Part model, mm, in its own coordinate system. A direction names the side the tool comes from. Round coordinates to 2 decimals unless told otherwise and drop trailing zeros. Loops run counter-clockwise (first coordinate to the right, second up) from the corner with the lowest first, then second, coordinate; pieces in that order, holes last. Notation, with made-up numbers: M 63.5,67 L 94.5,67 A21 ccw 94.5,106 Z; hole C -35.75,5.25 d2. An arc over 180 degrees is marked long. Put each result on its own line as item: value. Start each with the question number.
1) Pull direction Y, two halves, no side cores. Call faces 6 (the cylindrical face through (-0.495, -97.905, 0.21)), 7 (the cylindrical face through (-8.337, -54.779, -3.07)), 8 (the flat face through (26, -105.4, 0)): +Y half, -Y half, draft (parallel to the pull), parting line (faces both ways), or undercut.
2) Slice it at A-A on y = 0. Give the cut face in (x, z).
3) Probe line 1 along Y through (x, z) = (0.5, 5.5); line 2 along Y through (x, z) = (1, 8); line 3 along Z through (x, y) = (-30, -117). List the from-to ranges inside material, lowest first.
4) Drop flat-ended pins along their axis: pin 1 Ø16 at (x, y) = (-3.5, -47) entering from -Z; pin 2 Ø6 at (x, y) = (1.5, -45.5) entering from +Z; pin 3 Ø1.5 at (y, z) = (-23, 6.5) entering from +X; pin 4 Ø11 at (x, y) = (0, 0) entering from +Z. Give the stop position or say it passes through.
5) Which spindle directions (+Z, -Z, +X, -X, +Y, -Y) get a long thin tool onto all of the face, cutting with end or side? Do faces 1 (the flat face through (30, -117.4, 9)), 2 (the flat face through (-30, -117.4, 9)), 3 (the cylindrical face through (9.444, -53.631, 6.93)), 4 (the cylindrical face through (-35, -111, 0)), 5 (the flat face through (0, -62, -2.5)). Say none if no direction does.
```python
from build123d import *

# Parameters (mm, degrees)
SKETCH2_R           = 12.5
SKETCH2_R_2         = 9
BOSS_EXTRUDE1_DEPTH = 10
BOSS_EXTRUDE2_DEPTH = 15
BOSS_EXTRUDE3_DEPTH = 7.5
CUT_EXTRUDE2_START  = 7.5
CUT_EXTRUDE2_DEPTH  = 5
BOSS_EXTRUDE8_REACH = 149.366
BOSS_EXTRUDE8_START = 12
SKETCH4_R           = 3.25
SKETCH4_14_R        = 3.25
CUT_EXTRUDE3_DEPTH  = 136.366207009
FILLET1_R           = 2
FILLET5_R           = 2


with BuildPart() as part:
    # Sketch2 → Boss-Extrude1 (new, symmetric)
    with BuildSketch(Plane.XY):
        Circle(SKETCH2_R)
        Circle(SKETCH2_R_2, mode=Mode.SUBTRACT)
    extrude(amount=BOSS_EXTRUDE1_DEPTH, both=True)



with BuildPart() as body_2:
    # Sketch2_3 → Boss-Extrude2 (new, symmetric)
    with BuildSketch(Plane.XY):
        with BuildLine():
            ThreePointArc((15.952867936, -100.506382817), (8.454666221, -96.342389581), (0, -94.9))
            Line((0, -94.9), (0, -97.9))
            ThreePointArc((0, -97.9), (15.909902577, -104.490097423), (22.5, -120.4))
            Line((22.5, -120.4), (35, -120.4))
            Line((35, -120.4), (35, -117.4))
            Line((35, -117.4), (25.322914524, -117.4))
            ThreePointArc((25.322914524, -117.4), (22.299576897, -108.031537274), (15.952867936, -100.506382817))
        make_face()
        with BuildLine():
            Line((0, -97.9), (0, -94.9))
            ThreePointArc((0, -94.9), (-8.454666221, -96.342389581), (-15.952867936, -100.506382817))
            ThreePointArc((-15.952867936, -100.506382817), (-22.299576897, -108.031537274), (-25.322914524, -117.4))
            Line((-25.322914524, -117.4), (-35, -117.4))
            Line((-35, -117.4), (-35, -120.4))
            Line((-35, -120.4), (-22.5, -120.4))
            ThreePointArc((-22.5, -120.4), (-15.909902577, -104.490097423), (0, -97.9))
        make_face()
    extrude(amount=BOSS_EXTRUDE2_DEPTH, both=True)


with BuildPart() as part_1:
    add(part.part)

    add(body_2.part)  # Boss-Extrude3 merges body 2
    # Sketch2_4 → Boss-Extrude3 (add, symmetric)
    with BuildSketch(Plane.XY):
        with BuildLine():
            Line((0, -94.9), (0, -12.5))
            ThreePointArc((0, -12.5), (-4.253905297, -11.753905297), (-8, -9.604686356))
            Line((-8, -9.604686356), (-15.952867936, -100.506382817))
            ThreePointArc((-15.952867936, -100.506382817), (-8.454666221, -96.342389581), (0, -94.9))
        make_face()
        with BuildLine():
            ThreePointArc((8, -9.604686356), (4.253905297, -11.753905297), (0, -12.5))
            Line((0, -12.5), (0, -94.9))
            ThreePointArc((0, -94.9), (8.454666221, -96.342389581), (15.952867936, -100.506382817))
            Line((15.952867936, -100.506382817), (8, -9.604686356))
        make_face()
    extrude(amount=BOSS_EXTRUDE3_DEPTH, both=True)

    # Sketch3 → Cut-Extrude2 (cut)
    with BuildSketch(Plane.XY.offset(CUT_EXTRUDE2_START)):
        with BuildLine():
            Line((-5.4187458, -14.521955583), (-12.438451255, -94.757556076))
            ThreePointArc((-12.438451255, -94.757556076), (0, -91.9), (12.438451255, -94.757556076))
            Line((12.438451255, -94.757556076), (5.4187458, -14.521955583))
            ThreePointArc((5.4187458, -14.521955583), (0, -15.5), (-5.4187458, -14.521955583))
        make_face()
    cut_extrude2 = extrude(amount=-CUT_EXTRUDE2_DEPTH, mode=Mode.SUBTRACT)

    # Mirror1: Cut-Extrude2 across plane
    add(cut_extrude2.mirror(Plane.XY), mode=Mode.SUBTRACT)

    # Sketch4 → Boss-Extrude8 (add, up to next)
    with BuildSketch(Plane(origin=(0, -117.4, 0), x_dir=(1, 0, 0), z_dir=(0, 1, 0)).offset(BOSS_EXTRUDE8_START), mode=Mode.PRIVATE) as boss_extrude8_sk1:
        with BuildLine():
            Line((30, 5.019595967), (18, 5.019595967))
            Line((18, 5.019595967), (18, -4.980404033))
            Line((18, -4.980404033), (30, -4.980404033))
            ThreePointArc((30, -4.980404033), (35, 0.019595967), (30, 5.019595967))
        make_face()
        with Locations((30, 0.019595967)):
            Circle(SKETCH4_R, mode=Mode.SUBTRACT)
    boss_extrude8_tool1 = extrude(boss_extrude8_sk1.sketch, amount=-BOSS_EXTRUDE8_REACH, mode=Mode.PRIVATE) - part_1.part
    boss_extrude8 = boss_extrude8_tool1.solids().sort_by_distance((24.95057, -105.4, -0.019596))[0]
    add(boss_extrude8)

    # Sketch4_14 → Cut-Extrude3 (cut, symmetric)
    with BuildSketch(Plane(origin=(0, -117.4, 0), x_dir=(1, 0, 0), z_dir=(0, 1, 0))):
        with Locations(Location((30, 0.019595967, 0), (0, 0, 270))):
            Circle(SKETCH4_14_R)
    cut_extrude3 = extrude(amount=CUT_EXTRUDE3_DEPTH, both=True, mode=Mode.SUBTRACT)

    # Mirror2: Boss-Extrude8, Cut-Extrude3 across plane
    add(boss_extrude8.mirror(Plane(origin=(0, 0, 0), x_dir=(0, 0, 1), z_dir=(1, 0, 0))))
    add(cut_extrude3.mirror(Plane(origin=(0, 0, 0), x_dir=(0, 0, 1), z_dir=(1, 0, 0))), mode=Mode.SUBTRACT)

    # Fillet1
    fillet1_edges = [part_1.edges().sort_by_distance(p)[0] for p in [
        (0, -91.9, -7.5),
        (-12.438451255, -94.757556076, -5),
        (8.928598527, -54.63975583, -7.5),
        (12.438451255, -94.757556076, -5),
        (0, -15.5, -7.5),
        (5.4187458, -14.521955583, -5),
        (-8.928598527, -54.63975583, -7.5),
        (-5.4187458, -14.521955583, -5),
        (0, -91.9, -2.5),
        (8.928598527, -54.63975583, -2.5),
        (0, -15.5, -2.5),
        (-8.928598527, -54.63975583, -2.5),
    ]]
    fillet(fillet1_edges, radius=FILLET1_R)

    # Fillet5
    fillet5_edges = [part_1.edges().sort_by_distance(p)[0] for p in [
        (0, -91.9, 2.5),
        (12.438451255, -94.757556076, 5),
        (-8.928598527, -54.63975583, 2.5),
        (-12.438451255, -94.757556076, 5),
        (0, -15.5, 2.5),
        (-5.4187458, -14.521955583, 5),
        (8.928598527, -54.63975583, 2.5),
        (5.4187458, -14.521955583, 5),
        (0, -91.9, 7.5),
        (8.928598527, -54.63975583, 7.5),
        (0, -15.5, 7.5),
        (-8.928598527, -54.63975583, 7.5),
    ]]
    fillet(fillet5_edges, radius=FILLET5_R)


solid = part_1.part
```
Recorded:
1. face 6: -Y half
1. face 7: undercut
1. face 8: +Y half
2. outline: M -12.5,-10 L -9,-10 L -9,10 L -12.5,10 Z; M 9,-10 L 12.5,-10 L 12.5,10 L 9,10 Z
3. line 1: y = -97.91 to -91.9, -15.49 to -8.99, 8.99 to 12.49
3. line 2: y = -97.92 to -94.92, -12.46 to -8.94, 8.94 to 12.46
3. line 3: z = -5.02 to -3.27, 3.23 to 4.98
4. pin 1: stops at z = -7.5
4. pin 2: stops at z = 2.5
4. pin 3: stops at x = 9.24
4. pin 4: passes through
5. face 1: +Z, +X, +Y
5. face 2: +Z, -X, +Y
5. face 3: +Z
5. face 4: -X, +Y
5. face 5: -Z
